Autodesk Inventor part; units mm, degrees
ref_plane "YZ Plane" through (0, 0, 0) normal (1, 0, 0) x (0, 1, 0)
ref_plane "XZ Plane" through (0, 0, 0) normal (0, 1, 0) x (-1, 0, 0)
ref_plane "XY Plane" through (0, 0, 0) normal (0, 0, 1) x (1, 0, 0)
sketch "Sketch1" plane through (0, 0, 0) normal (0, 0, 1) x (1, 0, 0)
  line L0 (-19.05, -20) -> (-60.1594, -68.9923)
  line L1 (-6.35, -7.3) -> (0, -7.3)
  line L2 (0, -7.3) -> (0, -13.65)
  line L3 (0, -13.65) -> (-6.35, -13.65)
  line L4 (-6.35, -13.65) -> (-6.35, -7.3)
  line L5 (6.35, -4.953) -> (0, -4.953)
  line L6 (0, -4.953) -> (0, 4.953)
  line L7 (0, 4.953) -> (6.35, 4.953)
  line L8 (6.35, 4.953) -> (6.35, -4.953)
  line L9 (-6.35, 13.65) -> (0, 13.65)
  line L10 (0, 13.65) -> (0, 7.3)
  line L11 (0, 7.3) -> (-6.35, 7.3)
  line L12 (-6.35, 7.3) -> (-6.35, 13.65)
  line L13 (0, -20) -> (-19.05, -20)
  line L14 (-19.05, -20) -> (-19.05, 20)
  line L15 (-19.05, 20) -> (0, 20)
  line L16 (0, 20) -> (0, -20)
  line L17 (-48.9804, -78.3726) -> (-8.1634, -29.7288)
  line L18 (-8.1634, -29.7288) -> (0, -20)
  line L19 (-48.9804, -78.3726) -> (-60.1594, -68.9923)
  line L20 (-56.0777, -64.1279) -> (-51.996, -59.2635)
  line L21 (-51.996, -59.2635) -> (-56.8604, -55.1818)
  line L22 (-56.8604, -55.1818) -> (-60.9421, -60.0462)
  line L23 (-60.9421, -60.0462) -> (-56.0777, -64.1279)
  line L24 (-47.9143, -54.3991) -> (-43.8326, -49.5348)
  line L25 (-43.8326, -49.5348) -> (-48.697, -45.4531)
  line L26 (-48.697, -45.4531) -> (-52.7787, -50.3174)
  line L27 (-52.7787, -50.3174) -> (-47.9143, -54.3991)
  line L28 (-39.7509, -44.6704) -> (-35.6692, -39.806)
  line L29 (-35.6692, -39.806) -> (-40.5336, -35.7243)
  line L30 (-40.5336, -35.7243) -> (-44.6153, -40.5887)
  line L31 (-44.6153, -40.5887) -> (-39.7509, -44.6704)
  arc A0 (-48.9804, -78.3726) -> (0, -20) centre (-59.2731, -20) ccw
  point P0 (0, 0)
  point P1 (0, 0)
  dimension "d0" = 6.35
  dimension "d2" = 9.906
  dimension "d3" = 40
  dimension "d4" = 6.35
  dimension "d5" = 6.35
  dimension "d6" = 6.35
  dimension "d10" = 50
  dimension "d11" = 19.05
  dimension "d12" = 12.7
  dimension "d15" = 6.35
  dimension "d16" = 6.35
  dimension "d19" = 12.7
  dimension "d24" = 76.2
extrude "Extrusion1" add sketch "Sketch1" along normal blind 6.35 contours L13 L18 L17 L19 L0 | L14 L15 L16 L9 L12 L11 L6 L1 L4 L3 L13 | L0 L31 L30 L29 | A0 L17 L18 | L0 L27 L26 L25 | L6 L7 L8 L5 | L23 L22 L21 L0
properties part number "acrylic kinect bracket - bracket"
Can you work these out from the model? Positions are in its coordinate system, mm. A direction names the side the tool comes from. Coordinates: 2 decimals unless noted, no trailing zeros. Order: outer loops, then holes, each group sorted by start corner. A loop starts at its lowest first (then second) coordinate and runs counter-clockwise, first axis right, second up. Notation, with made-up numbers: (60.5, 64.5) - (104.5, 64.5) arc R28 cw to (104.5, 102.5) - close; hole circle Ø4 at (89, 43.25). An arc over 180 degrees is marked (long way). Answer in a Markdown table with one row per item.
1. For pin 1 (1.5 mm diameter, centred on x = -41, z = 4.5, fed in from +Y); pin 2 (3 mm diameter, centred on y = 16, z = 3.5, fed in from +X); pin 3 (3 mm diameter, centred on x = -3, z = 3, fed in from -Y), each with a flat end and sliding along its axis, tell me the tip position at first contact or that it passes through.
Reply:
| item | result |
|---|---|
| pin 1 | stops at y = -35.72 |
| pin 2 | stops at x = 0 |
| pin 3 | stops at y = -42.65 |
2. If I drill on line 1 along X through (y, z) = (-14.5, 5.75); line 2 along X through (y, z) = (-57, 4.75); line 3 along X through (y, z) = (-3.5, 0.75), over which ranges is the centre line in solid material (lowest first)?
Reply:
| item | result |
|---|---|
| line 1 | x = -19.05 to 0 |
| line 2 | x = -58.39 to -54.69, -50.1 to -12.97 |
| line 3 | x = -19.05 to 6.35 |
3. For faces 1 (the flat face through (3, 4.953, 3)), 2 (the flat face through (-58.54, -62.06, 3.13)), 3 (the flat face through (-6.35, -11, 3)), 4 (the flat face through (-46.231, -47.523, 3.131)), 5 (the flat face through (0, -6, 3)), which set-ups out of +Z, -Z, +X, -X, +Y, -Y let a thin tool reach every point of the face, with its end or its side?
Reply:
| item | result |
|---|---|
| face 1 | +Z, -Z, +X, +Y |
| face 2 | +Z, -Z, -X |
| face 3 | +Z, -Z, +X |
| face 4 | +Z, -Z |
| face 5 | +Z, -Z, +X, -Y |
4. Suppose I cut it at B-B (x = -5). Please give me the cut outline in (y, z), and give its area (3 significant figures).
Reply:
| item | result |
|---|---|
| outline | (-43.83, 0) - (-13.65, 0) - (-13.65, 6.35) - (-43.83, 6.35) - close; (-7.3, 0) - (7.3, 0) - (7.3, 6.35) - (-7.3, 6.35) - close; (13.65, 0) - (20, 0) - (20, 6.35) - (13.65, 6.35) - close |
| area | 325 mm^2 |
5. Suppose I cut it at A-A (y = -56.5). Please give me the cut outline in (x, z), and give its area (3 significant figures).
Reply:
| item | result |
|---|---|
| outline | (-57.97, 0) - (-55.29, 0) - (-55.29, 6.35) - (-57.97, 6.35) - close; (-49.68, 0) - (-12.57, 0) - (-12.57, 6.35) - (-49.68, 6.35) - close |
| area | 253 mm^2 |
6. If we mould it in two halves opening along Y, with no side actions, what happens to faces 6 (the flat face through (-10, 20, 3)), 7 (the flat face through (-6.35, 10, 3)), 8 (the flat face through (-3, 7.3, 3)), 9 (the flat face through (-28, -39, 0))? For each: pulls with the +Y half, pulls with the -Y half, needs draft (parallel to the pull), parting line crosses it, or undercut.
Reply:
| item | result |
|---|---|
| face 6 | pulls with the +Y half |
| face 7 | undercut |
| face 8 | undercut |
| face 9 | needs draft |
7. Suppose I cut it at C-C (y = -17). Please give me the cut outline in (x, z), and give its area (3 significant figures).
Reply:
| item | result |
|---|---|
| outline | (-19.05, 0) - (0, 0) - (0, 6.35) - (-19.05, 6.35) - close |
| area | 121 mm^2 |
